Print and shaded views of the part. All mm, measured from the part's lowest x, y and z. Give positions to 0.01 mm unless a question says otherwise; leave off trailing zeros. Order: outer loops, then holes, each group sorted by start corner. A loop starts at its lowest first (then second) coordinate and runs counter-clockwise, first axis right, second up. Notation, with made-up numbers: (-18.5, -27.5) -> (31.5, -27.5) arc R17 ccw to (31.5, -9.5) -> close; hole circle Ø11 at (-23.75, -17). An arc over 180 degrees is marked (long way). One line per question, with ' | ' between items. Start each with the question number.
(1) Cut at B-B (z = 0.45). Give the cut face in (x, y).
(2) Cut at A-A (y = 3.6). Give the cut face in (x, z).
(3) Cut at D-D (x = 1). Give the cut face in (y, z).
(4) Pull direction X, two halves, no side cores. Call the marked faces 1, 2, 3 and 4: +X half, -X half, draft (parallel to the pull), parting line (faces both ways), or undercut.
(5) Drill centre lines: L1, parallel to X at y = 5, z = 0.1; L2, parallel to Y at x = 3.25, z = 0.4. Where is each one in solid material? Low to high. Write a range as from..to.
(6) Cut at C-C (y = 0.6). Give the cut face in (x, z).
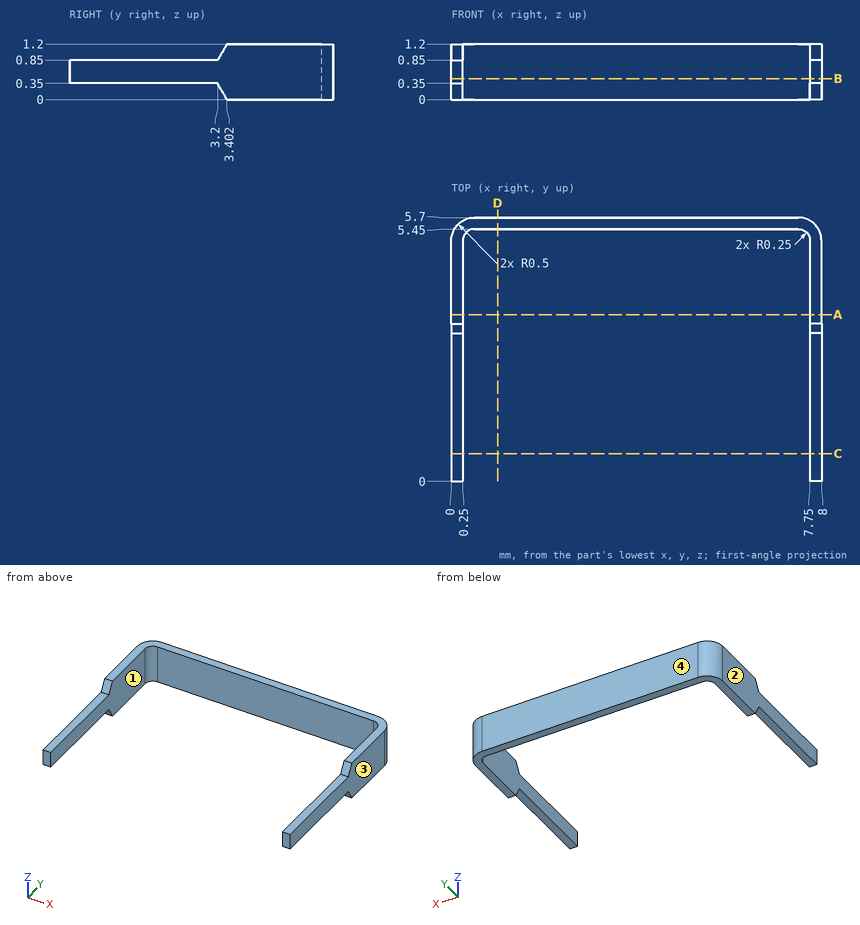
Result set:
1) outline: (0, 0) -> (0.25, 0) -> (0.25, 5.2) arc R0.25 cw to (0.5, 5.45) -> (7.5, 5.45) arc R0.25 cw to (7.75, 5.2) -> (7.75, 0) -> (8, 0) -> (8, 5.2) arc R0.5 ccw to (7.5, 5.7) -> (0.5, 5.7) arc R0.5 ccw to (0, 5.2) -> close
2) outline: (0, 0) -> (0.25, 0) -> (0.25, 1.2) -> (0, 1.2) -> close; (7.75, 0) -> (8, 0) -> (8, 1.2) -> (7.75, 1.2) -> close
3) outline: (5.45, 0) -> (5.7, 0) -> (5.7, 1.2) -> (5.45, 1.2) -> close
4) face 1: undercut | face 2: -X half | face 3: +X half | face 4: draft
5) L1: x = 0..0.25, 7.75..8 | L2: y = 5.45..5.7
6) outline: (0, 0.35) -> (0.25, 0.35) -> (0.25, 0.85) -> (0, 0.85) -> close; (7.75, 0.35) -> (8, 0.35) -> (8, 0.85) -> (7.75, 0.85) -> close
